Drawing for the job (mm, zero at the part's lowest x, y, z). Round coordinates to 2 decimals unless told otherwise and drop trailing zeros. Write each loop counter-clockwise with the first axis right and the second up, starting at its lowest first coordinate (ties: lowest second). Pieces come first, ordered by that corner, then holes.
Item 1: Band-saw the part on C-C, the plane y = 1.65. Write the cut outline in (x, z), then the cut area to 3 significant figures.
Item 2: Band-saw the part on B-B, the plane x = 16. Write the cut outline in (y, z).
Item 3: Drop a flat-ended pin along its axis: pin 1 Ø1.5 at (x, y) = (53.5, 1.5) entering from -Z. Give the stop position or say it passes through.
Item 4: Band-saw the part on A-A, the plane z = 47. Write the cut outline in (x, y).
Item 5: Wall check: probe 1 along Z at (x, y) = (18.5, 1.05); probe 2 along Z at (x, y) = (24, 0.5). Give the ranges that are in metal, low to high.
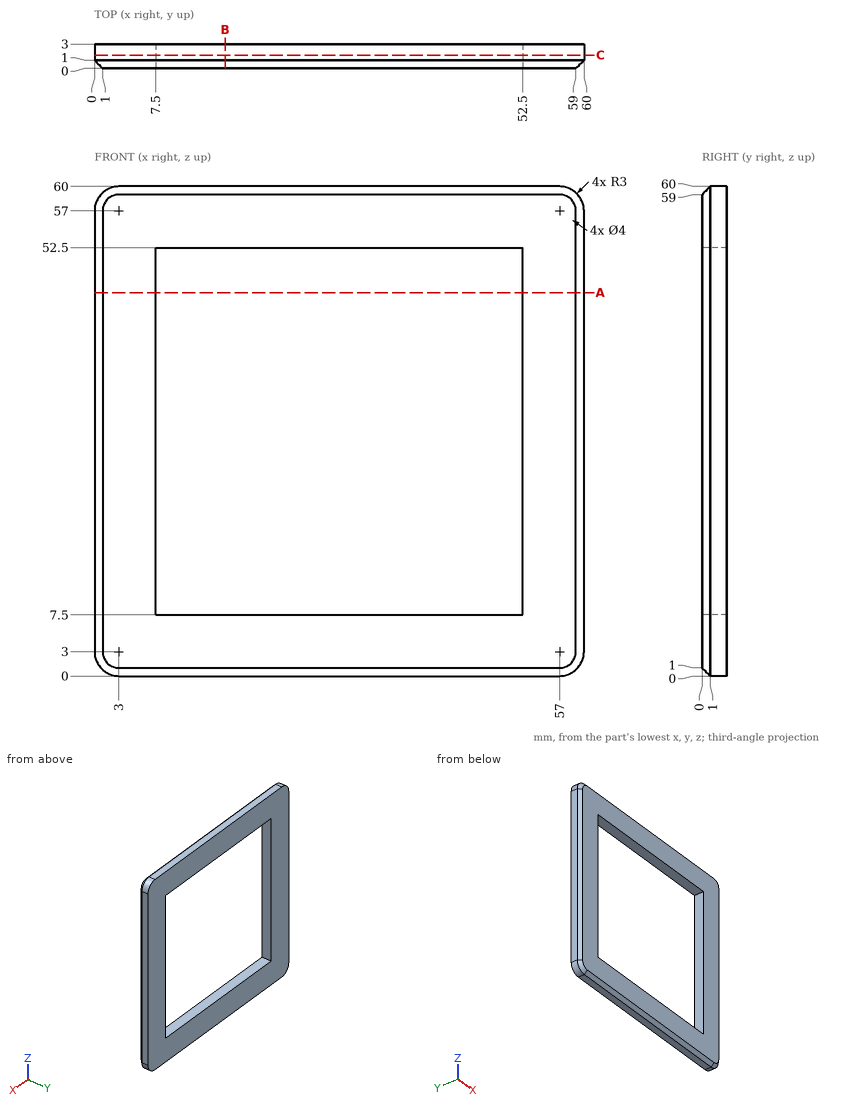
Results:
1. outline: (0, 3) arc R3 ccw to (3, 0) - (57, 0) arc R3 ccw to (60, 3) - (60, 57) arc R3 ccw to (57, 60) - (3, 60) arc R3 ccw to (0, 57) - close; hole (7.5, 7.5) - (52.5, 7.5) - (52.5, 52.5) - (7.5, 52.5) - close
1. area: 1,570 mm2
2. outline: (0, 1) - (1, 0) - (3, 0) - (3, 7.5) - (0, 7.5) - close; (0, 52.5) - (3, 52.5) - (3, 60) - (1, 60) - (0, 59) - close
3. pin 1: stops at z = 0
4. outline: (0, 1) - (1, 0) - (7.5, 0) - (7.5, 3) - (0, 3) - close; (52.5, 0) - (59, 0) - (60, 1) - (60, 3) - (52.5, 3) - close
5. probe 1: z = 0 to 7.5, 52.5 to 60
5. probe 2: z = 0.5 to 7.5, 52.5 to 59.5
